from build123d import *
from build123d.topology import SkipClean

# Parameters (mm, degrees)
SKETCH1_R           = 8.33
BOSS_EXTRUDE1_DEPTH = 7.16
SKETCH2_R           = 3.5
BOSS_EXTRUDE2_DEPTH = 8.5
BOSS_EXTRUDE6_START = -8.5
SKETCH6_R           = 3
BOSS_EXTRUDE6_DEPTH = 27
SKETCH7_W           = 6
SKETCH7_H           = 1
CUT_EXTRUDE1_DEPTH  = 16.5
SKETCH3_W           = 15
SKETCH3_H           = 11.20454244
BOSS_EXTRUDE3_DEPTH = 1.2
BOSS_EXTRUDE4_START = -0.2
SKETCH4_W           = 1.15
SKETCH4_H           = 4.9
BOSS_EXTRUDE4_DEPTH = 0.6
LPATTERN1_COUNT     = 2
LPATTERN1_PITCH     = 5
LPATTERN1_COL_COUNT = 2
LPATTERN1_COL_PITCH = 5
BOSS_EXTRUDE5_DEPTH = 4


with BuildPart() as part:
    # Sketch1 → Boss-Extrude1 (new body)
    with BuildSketch(Plane.XY):
        with Locations(Location((0, 0, 0), (0, 0, 180))):
            Circle(SKETCH1_R)
    extrude(amount=BOSS_EXTRUDE1_DEPTH)

    # Sketch2 → Boss-Extrude2 (add)
    with BuildSketch(Plane.XY.offset(7.16)):
        Circle(SKETCH2_R)
    extrude(amount=BOSS_EXTRUDE2_DEPTH)

    # Sketch6 → Boss-Extrude6 (add)
    with BuildSketch(Plane.XY.offset(15.66).offset(BOSS_EXTRUDE6_START)):
        Circle(SKETCH6_R)
    extrude(amount=BOSS_EXTRUDE6_DEPTH)

    # Sketch7 → Cut-Extrude1 (cut)
    with BuildSketch(Plane.XY.offset(34.16)):
        Rectangle(SKETCH7_W, SKETCH7_H)
    extrude(amount=-CUT_EXTRUDE1_DEPTH, mode=Mode.SUBTRACT)

    # Sketch3 → Boss-Extrude3 (add)
    with BuildSketch(Plane.XY.offset(7.16)):
        with Locations((0, -6.09772878)):
            Rectangle(SKETCH3_W, SKETCH3_H)
    extrude(amount=-BOSS_EXTRUDE3_DEPTH)

    # Sketch4 → Boss-Extrude4 (add)
    with BuildSketch(Plane(origin=(0, 0, 5.96), x_dir=(-1, 0, 0), z_dir=(0, 0, -1)).offset(BOSS_EXTRUDE4_START)):
        with Locations((0, -14.15)):
            Rectangle(SKETCH4_W, SKETCH4_H)
    boss_extrude4 = extrude(amount=BOSS_EXTRUDE4_DEPTH)

    # LPattern1: Boss-Extrude4 ×2
    with Locations(*[(i * LPATTERN1_PITCH, 0, 0) for i in range(1, LPATTERN1_COUNT)]):
        add(boss_extrude4)

    # LPattern1 col: Boss-Extrude4 ×2
    with Locations(*[(-i * LPATTERN1_COL_PITCH, 0, 0) for i in range(1, LPATTERN1_COL_COUNT)]):
        add(boss_extrude4)

    # Sketch5 → Boss-Extrude5 (add)
    with SkipClean():  # the faces are left unmerged after this step: merging them gives an invalid solid
        with BuildSketch(Plane.XY.offset(7.16)):
            with BuildLine():
                Line((-8.219878345, 1.35), (-6.937064197, 1.139315726))
                ThreePointArc((-6.937064197, 1.139315726), (-7.03, 0), (-6.937064197, -1.139315726))
                Line((-6.937064197, -1.139315726), (-8.219878345, -1.35))
                ThreePointArc((-8.219878345, -1.35), (-8.33, 0), (-8.219878345, 1.35))
            make_face()
        extrude(amount=BOSS_EXTRUDE5_DEPTH)
    add(part.part.scale(1), mode=Mode.REPLACE)  # the faces are merged on a copy


solid = part.part
Geometry check sheet. Reference: the model listing, model coordinates, mm. A direction names the side the tool comes from. Round coordinates to 2 decimals unless told otherwise and drop trailing zeros. Order: outer loops, then holes, each group sorted by start corner. A loop starts at its lowest first (then second) coordinate and runs counter-clockwise, first axis right, second up. Notation, with made-up numbers: (10.25, 10.25) - (31.25, 10.25) arc R18 ccw to (31.25, 23.25) - close; hole circle Ø4 at (76, 33). An arc over 180 degrees is marked (long way). One line per question, with ' | ' between items. Start each with the question number.
(1) Depth check by flat-ended pin: pin 1 Ø6 at (y, z) = (-1, 19) entering from +X; pin 2 Ø1.1 at (x, y) = (-1.5, 0) entering from +Z; pin 3 Ø0.5 at (y, z) = (-13, 6) entering from -X (3 decimals); pin 4 Ø3 at (y, z) = (2.5, 16) entering from -X. Enter the tip coordinate at first touch or a pass-through.
(2) Release check for a two-part mould opening along X. For faces 1 (the flat face through (0, 0, 17.66)), 2 (the flat face through (-7.587, 1.246, 9.132)), 3 (the flat face through (7.5, -8, 7)) record: released by +X, released by -X, zero draft, split by the parting line, or undercut.
(3) Access from +Z, -Z, +X, -X, +Y, -Y to the whole of each face (thin tool, end or side, straight path). Record for faces 4 (the flat face through (-7.569, -1.243, 9.132)), 5 (the flat face through (-5, -14, 6.16)), 6 (the flat face through (-7.5, -8, 7)).
(4) Sectioned sample at C-C on x = 0. Record the cut outline in (y, z), and give its area (3 significant figures).
(5) Sectioned sample at A-A on y = -14. Record the cut outline in (x, z) (3 decimals), and give its area (3 significant figures).
(6) Sectioned sample at D-D on y = 0. Record the cut outline in (x, z).
(7) Thickness scan on L1, parallel to Z at x = -1.5, y = 3.5; L2, parallel to Z at x = 7, y = -6.5; L3, parallel to Y at x = 1.75, z = 24. Record the ranges inside material, lowest first. Write a range as [from, to].
(8) Sectioned sample at B-B on z = 10.5. Record the cut outline in (x, y).
Conclusion:
1) pin 1: stops at x = 3 | pin 2: stops at z = 34.16 | pin 3: stops at x = -5.575 | pin 4: stops at x = -3.34
2) face 1: zero draft | face 2: undercut | face 3: released by +X
3) face 4: +Z, -Y | face 5: +Z, +X, -X, -Y | face 6: +Z, -Z, -X, -Y
4) outline: (-16.6, 5.56) - (-11.7, 5.56) - (-11.7, 5.96) - (-8.33, 5.96) - (-8.33, 0) - (8.33, 0) - (8.33, 7.16) - (3.5, 7.16) - (3.5, 15.66) - (3, 15.66) - (3, 34.16) - (0.5, 34.16) - (0.5, 17.66) - (-0.5, 17.66) - (-0.5, 34.16) - (-3, 34.16) - (-3, 15.66) - (-3.5, 15.66) - (-3.5, 7.16) - (-11.7, 7.16) - (-11.7, 6.16) - (-16.6, 6.16) - close | area: 280 mm2
5) outline: (-5.575, 5.56) - (-4.425, 5.56) - (-4.425, 6.16) - (-5.575, 6.16) - close; (-0.575, 5.56) - (0.575, 5.56) - (0.575, 6.16) - (-0.575, 6.16) - close; (4.425, 5.56) - (5.575, 5.56) - (5.575, 6.16) - (4.425, 6.16) - close | area: 2.07 mm2
6) outline: (-8.33, 0) - (8.33, 0) - (8.33, 7.16) - (3.5, 7.16) - (3.5, 15.66) - (3, 15.66) - (3, 17.66) - (-3, 17.66) - (-3, 15.66) - (-3.5, 15.66) - (-3.5, 7.16) - (-7.03, 7.16) - (-7.03, 11.16) - (-8.33, 11.16) - close
7) L1: z = [0, 7.16] | L2: z = [5.96, 7.16] | L3: y = [-2.44, -0.5], [0.5, 2.44]
8) outline: (-8.22, -1.35) - (-6.94, -1.14) arc R7.03 cw to (-6.94, 1.14) - (-8.22, 1.35) arc R8.33 ccw to start; circle Ø7 at (0, 0)
